Geometry: final body of the model. Coordinates: model frame, mm. Give positions to 0.01 mm unless a question says otherwise; leave off trailing zeros. Loops run counter-clockwise (first coordinate to the right, second up) from the corner with the lowest first, then second, coordinate; pieces in that order, holes last. Notation, with made-up numbers: (-35, 80) - (-15, 80) arc R27 ccw to (-15, 101) - close; hole circle Ø4 at (-37.5, -32.5). An arc over 180 degrees is marked (long way). Answer in a Markdown table with one row per item.
from build123d import *

# Parameters (mm, degrees)
SKETCH2_R           = 2.032
SKETCH2_R_2         = 4.318
BOSS_EXTRUDE1_DEPTH = 2.54


with BuildPart() as part:
    # Sketch2 → Boss-Extrude1 (new body)
    with BuildSketch(Plane(origin=(0, 0, 0), x_dir=(1, 0, 0), z_dir=(0, 1, 0))):
        with BuildLine():
            ThreePointArc((56.007, 12.7), (68.707, 0), (56.007, -12.7))
            Line((56.007, -12.7), (-8.001, -12.7))
            ThreePointArc((-8.001, -12.7), (-20.701, 0), (-8.001, 12.7))
            Line((-8.001, 12.7), (56.007, 12.7))
        make_face()
        with Locations(Location((48.006, 8.001, 0), (0, 0, 270))):
            Circle(SKETCH2_R, mode=Mode.SUBTRACT)
        with Locations(Location((56.007, 0, 0), (0, 0, 270))):
            Circle(SKETCH2_R, mode=Mode.SUBTRACT)
        with Locations(Location((48.006, 0, 0), (0, 0, 270))):
            Circle(SKETCH2_R_2, mode=Mode.SUBTRACT)
        with Locations(Location((48.006, -8.001, 0), (0, 0, 270))):
            Circle(SKETCH2_R, mode=Mode.SUBTRACT)
        with Locations(Location((32.004, 8.001, 0), (0, 0, 270))):
            Circle(SKETCH2_R, mode=Mode.SUBTRACT)
        with Locations(Location((40.005, 0, 0), (0, 0, 270))):
            Circle(SKETCH2_R, mode=Mode.SUBTRACT)
        with Locations(Location((32.004, 0, 0), (0, 0, 270))):
            Circle(SKETCH2_R_2, mode=Mode.SUBTRACT)
        with Locations(Location((32.004, -8.001, 0), (0, 0, 270))):
            Circle(SKETCH2_R, mode=Mode.SUBTRACT)
        with Locations(Location((16.002, 8.001, 0), (0, 0, 270))):
            Circle(SKETCH2_R, mode=Mode.SUBTRACT)
        with Locations(Location((24.003, 0, 0), (0, 0, 270))):
            Circle(SKETCH2_R, mode=Mode.SUBTRACT)
        with Locations(Location((16.002, 0, 0), (0, 0, 270))):
            Circle(SKETCH2_R_2, mode=Mode.SUBTRACT)
        with Locations(Location((16.002, -8.001, 0), (0, 0, 270))):
            Circle(SKETCH2_R, mode=Mode.SUBTRACT)
        with Locations(Location((8.001, 0, 0), (0, 0, 270))):
            Circle(SKETCH2_R, mode=Mode.SUBTRACT)
        with Locations(Location((0, 8.001, 0), (0, 0, 270))):
            Circle(SKETCH2_R, mode=Mode.SUBTRACT)
        with Locations(Location((-8.001, 0, 0), (0, 0, 270))):
            Circle(SKETCH2_R, mode=Mode.SUBTRACT)
        with Locations(Location((0, -8.001, 0), (0, 0, 270))):
            Circle(SKETCH2_R, mode=Mode.SUBTRACT)
        with Locations(Location((0, 0, 0), (0, 0, 270))):
            Circle(SKETCH2_R_2, mode=Mode.SUBTRACT)
    extrude(amount=BOSS_EXTRUDE1_DEPTH)


solid = part.part
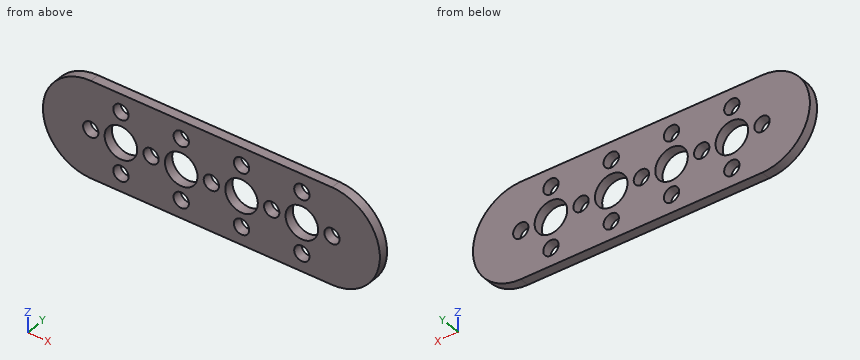
Q1. Material intervals for line 1 along Z through (x, y) = (48, 1.1); line 2 along X through (y, z) = (1.3, 6.5); line 3 along Z through (x, y) = (-1, 1.95), sorted ascending.
Check values:
| item | result |
|---|---|
| line 1 | -12.7 to -10.03, -5.97 to -4.32, 4.32 to 5.97, 10.03 to 12.7 |
| line 2 | -18.91 to -1.37, 1.37 to 14.63, 17.37 to 30.63, 33.37 to 46.64, 49.38 to 66.92 |
| line 3 | -12.7 to -9.77, -6.23 to -4.2, 4.2 to 6.23, 9.77 to 12.7 |
Q2. Cut plane A-A (x = 0). Output: boundary loops of the cut face in (y, z).
Check values:
| item | result |
|---|---|
| outline | (0, -12.7) - (2.54, -12.7) - (2.54, -10.03) - (0, -10.03) - close; (0, -5.97) - (2.54, -5.97) - (2.54, -4.32) - (0, -4.32) - close; (0, 4.32) - (2.54, 4.32) - (2.54, 5.97) - (0, 5.97) - close; (0, 10.03) - (2.54, 10.03) - (2.54, 12.7) - (0, 12.7) - close |
Q3. Cut plane B-B (z = 0). Give the number of separate pieces and of enclosed holes in the cut face, and give its area (3 significant figures).
Check values:
| item | result |
|---|---|
| separate pieces | 10 |
| enclosed holes | 0 |
| area | 87.7 mm² |
Q4. Cut plane D-D (x = 61.5). Output: boundary loops of the cut face in (y, z).
Check values:
| item | result |
|---|---|
| outline | (0, -11.45) - (2.54, -11.45) - (2.54, 11.45) - (0, 11.45) - close |
Q5. First-contact query: pin 1 (3.5 mm diameter, centred on x = 32.004, z = -8.001, fed in from +Y); pin 2 (1.5 mm diameter, centred on y = 2, z = 9, fed in from +X). Flat tips, straight axial feed; report the tip coordinate or a pass-through.
Check values:
| item | result |
|---|---|
| pin 1 | through |
| pin 2 | x = 65.66 |
